Solid Edge part; units mm, degrees
sketch "Sketch1" plane through (0, 0, 0) normal (0, 0, 1) x (1, 0, 0)
  line L0 (19.1, 20) -> (19.1, 15)
  line L1 (19.1, 15) -> (49.1, 15)
  line L2 (49.1, 15) -> (49.1, 20)
  line L3 (49.1, 20) -> (19.1, 20)
  line L4 (-7, -39.5) -> (-5, -39.5)
  line L5 (-5, -39.5) -> (-5, -14.5)
  line L6 (-5, -14.5) -> (-7, -14.5)
  line L7 (-7, -14.5) -> (-7, -39.5)
  line L8 (53.1, 43.5) -> (-53.1, 43.5)
  line L9 (-53.1, 43.5) -> (-53.1, -43.5)
  line L10 (-53.1, -43.5) -> (53.1, -43.5)
  line L11 (53.1, -43.5) -> (53.1, 43.5)
  line L12 (7, -39.5) -> (5, -39.5)
  line L13 (5, -39.5) -> (5, -14.5)
  line L14 (5, -14.5) -> (7, -14.5)
  line L15 (7, -14.5) -> (7, -39.5)
  line L16 (-49.1, 20) -> (-19.1, 20)
  line L17 (-19.1, 20) -> (-19.1, 15)
  line L18 (-19.1, 15) -> (-49.1, 15)
  line L19 (-49.1, 15) -> (-49.1, 20)
extrude "ExtrudedProtrusion_2" add sketch "Sketch1" along normal blind 10
sketch "Sketch2" plane through (0, 0, 10) normal (0, 0, 1) x (0, 1, 0)
  line L0 (41.5, -51.1) -> (-41.5, -51.1)
  line L1 (-41.5, -51.1) -> (-41.5, 51.1)
  line L2 (-41.5, 51.1) -> (41.5, 51.1)
  line L3 (41.5, 51.1) -> (41.5, -51.1)
  line L4 (-39.5, -7) -> (-39.5, -5)
  line L5 (-39.5, -5) -> (-14.5, -5)
  line L6 (-14.5, -5) -> (-14.5, -7)
  line L7 (-14.5, -7) -> (-39.5, -7)
  line L8 (15, 49.1) -> (20, 49.1)
  line L9 (20, 49.1) -> (20, 19.1)
  line L10 (20, 19.1) -> (15, 19.1)
  line L11 (15, 19.1) -> (15, 49.1)
  line L12 (-14.5, 5) -> (-14.5, 7)
  line L13 (-14.5, 7) -> (-39.5, 7)
  line L14 (-39.5, 7) -> (-39.5, 5)
  line L15 (-39.5, 5) -> (-14.5, 5)
  line L16 (15, -49.1) -> (20, -49.1)
  line L17 (20, -49.1) -> (20, -19.1)
  line L18 (20, -19.1) -> (15, -19.1)
  line L19 (15, -19.1) -> (15, -49.1)
extrude "ExtrudedCutout_1" cut sketch "Sketch2" against normal blind 7.9
sketch "Sketch3" plane through (0, 0, 10) normal (0, 0, 1) x (1, 0, 0)
  line L0 (-51.7, 42.1) -> (-51.7, -42.1)
  line L1 (-51.7, -42.1) -> (51.7, -42.1)
  line L2 (51.7, -42.1) -> (51.7, 42.1)
  line L3 (51.7, 42.1) -> (-51.7, 42.1)
  line L4 (53.1, 43.5) -> (-53.1, 43.5)
  line L5 (-53.1, 43.5) -> (-53.1, -43.5)
  line L6 (-53.1, -43.5) -> (53.1, -43.5)
  line L7 (53.1, -43.5) -> (53.1, 43.5)
extrude "ExtrudedCutout_2" cut sketch "Sketch3" against normal blind 1
sketch "Sketch4" plane through (0, 0, 2.1) normal (0, 0, 1) x (1, 0, 0)
  line L0 (-49.65, -5.6) -> (-49.65, 5.6)
  line L1 (-49.65, 5.6) -> (-51.1, 5.6)
  line L2 (-51.1, 5.6) -> (-51.1, -5.6)
  line L3 (-51.1, -5.6) -> (-49.65, -5.6)
extrude "ExtrudedProtrusion_3" add sketch "Sketch4" along normal blind 5
mirror "Mirror1" about plane through (0, 0, 0) normal (1, 0, 0) of "ExtrudedProtrusion_3"
sketch "Sketch5" plane through (-50.375, 0, 7.1) normal (0, 0, 1) x (0, 1, 0)
  line L0 (-2.4577, -0.725) -> (2.5423, -0.725)
  line L1 (2.5423, -0.725) -> (2.5423, 0.725)
  line L2 (2.5423, 0.725) -> (-2.4577, 0.725)
  line L3 (-2.4577, 0.725) -> (-2.4577, -0.725)
extrude "ExtrudedProtrusion_4" add sketch "Sketch5" along normal blind 8
mirror "Mirror2" about plane through (0, 0, 0) normal (1, 0, 0) of "ExtrudedProtrusion_4"
sketch "Sketch6" plane through (-50.375, -2.4577, 11.1) normal (0, -1, 0) x (0, 0, 1)
  line L0 (4, 2.675) -> (4, -0.725)
  line L1 (4, -0.725) -> (8, -0.725)
  line L2 (8, -0.725) -> (8, 0.675)
  line L3 (8, 0.675) -> (5, 2.675)
  line L4 (5, 2.675) -> (4, 2.675)
extrude "ExtrudedProtrusion_5" add sketch "Sketch6" against normal blind 5
mirror "Mirror3" about plane through (0, 0, 0) normal (1, 0, 0) of "ExtrudedProtrusion_5"
sketch "Sketch7" plane through (0, 0, 0) normal (0, 0, -1) x (0, 1, 0)
  line L0 (-4, 51.1) -> (4, 51.1)
  line L1 (4, 51.1) -> (4, 53.1)
  line L2 (4, 53.1) -> (-4, 53.1)
  line L3 (-4, 53.1) -> (-4, 51.1)
extrude "ExtrudedCutout_4" cut sketch "Sketch7" against normal blind 10
mirror "Mirror4" about plane through (0, 0, 0) normal (1, 0, 0) of "ExtrudedCutout_4"
sketch "Sketch8" plane through (0, 0, 2.1) normal (0, 0, 1) x (1, 0, 0)
  circle A0 centre (42.5, -25) radius 1.2
  circle A1 centre (42.5, -25) radius 2.4
  circle A2 centre (-42.5, -25) radius 2.4
  circle A3 centre (-42.5, -25) radius 1.2
  circle A4 centre (-42.5, 25) radius 1.2
  circle A5 centre (-42.5, 25) radius 2.4
  circle A6 centre (42.5, 25) radius 2.4
  circle A7 centre (42.5, 25) radius 1.2
extrude "ExtrudedProtrusion_6" add sketch "Sketch8" along normal blind 7.9
For this review, take the finished solid that the model builds, in its own axes (mm). A direction names the side the tool comes from. Coordinates: 2 decimals unless noted, no trailing zeros. Write each loop counter-clockwise with the first axis right and the second up, starting at its lowest first coordinate (ties: lowest second). Pieces come first, ordered by that corner, then holes. Notation, with made-up numbers: (51.25, 88.25) - (93.25, 88.25) arc R23 cw to (93.25, 109.25) - close; hole circle Ø3 at (-3.75, 43). An arc over 180 degrees is marked (long way). Put each result on its own line as item: value.
1. Add section A-A, the plane y = -32. Give the boundary of the cut face in (x, z), then the cut area to 3 significant figures.
Values found:
outline: (-53.1, 0) - (-7, 0) - (-7, 2.1) - (-51.1, 2.1) - (-51.1, 10) - (-51.7, 10) - (-51.7, 9) - (-53.1, 9) - close; (-5, 0) - (5, 0) - (5, 2.1) - (-5, 2.1) - close; (7, 0) - (53.1, 0) - (53.1, 9) - (51.7, 9) - (51.7, 10) - (51.1, 10) - (51.1, 2.1) - (7, 2.1) - close
area: 243 mm²
2. Wall thickness on probe 1 along Y at (x, z) = (42.5, 7.5); probe 2 along X at (y, z) = (2.5, 12); probe 3 along X at (y, z) = (20, 7.5): over which ranges is each line inside the solid? List them lowest first.
Values found:
probe 1: -43.5 to -41.5, -27.4 to -26.2, -23.8 to -22.6, 22.6 to 23.8, 26.2 to 27.4, 41.5 to 43.5
probe 2: -51.1 to -49.65, 49.65 to 51.1
probe 3: -53.1 to -51.1, 51.1 to 53.1
3. Mouldability with a two-part tool opening along X and no side actions: class faces 1 (the flat face through (-53.1, 24, 4)), 2 (the flat face through (-51.1, 22, 6)), 3 (the flat face through (51.1, 0, 6)) as released by +X, released by -X, zero draft, split by the parting line, or undercut.
Values found:
face 1: released by -X
face 2: undercut
face 3: released by +X
4. Add section B-B, the plane z = 4.5. Count the separate pieces of the cut face and the enclosed holes in it, then the cut area to 3 significant figures.
Values found:
separate pieces: 5
enclosed holes: 5
area: 812 mm²
5. For pin 1 (0.8 mm diameter, centred on y = -1, z = 16, fed in from +X); pin 2 (0.6 mm diameter, centred on x = -52, y = 0.5, fed in from -Z); pin 3 (1.2 mm diameter, centred on x = 50, y = -3.5, fed in from +Z), all flat-tipped, find the tip position at first contact; note any pin that passes through.
Values found:
pin 1: x = 53.05
pin 2: z = 15.1
pin 3: z = 7.1
6. Add section C-C, the plane x = -24. Give the boundary of the cut face in (y, z).
Values found:
outline: (-43.5, 0) - (15, 0) - (15, 2.1) - (-41.5, 2.1) - (-41.5, 10) - (-42.1, 10) - (-42.1, 9) - (-43.5, 9) - close; (20, 0) - (43.5, 0) - (43.5, 9) - (42.1, 9) - (42.1, 10) - (41.5, 10) - (41.5, 2.1) - (20, 2.1) - close
7. Machinability: for faces 4 (the cylindrical face through (43.61, -24.54, 5.99)), 5 (the flat face through (49.1, 17, 1)), 6 (the flat face through (-1, 1, 0)), which of the approach directions +Z, -Z, +X, -X, +Y, -Y give a long, thin tool a straight path to every point of the face, cutting with its end or side? Answer none if there is none.
Values found:
face 4: +Z
face 5: +Z, -Z
face 6: -Z, +X, -X, +Y, -Y
8. Add section D-D, the plane y = 34.5. Give the boundary of the cut face in (x, z).
Values found:
outline: (-53.1, 0) - (53.1, 0) - (53.1, 9) - (51.7, 9) - (51.7, 10) - (51.1, 10) - (51.1, 2.1) - (-51.1, 2.1) - (-51.1, 10) - (-51.7, 10) - (-51.7, 9) - (-53.1, 9) - close
